from build123d import *

# Parameters (mm, degrees)
F0_W     = 150
F0_H     = 150
F1_DEPTH = 2


with BuildPart() as f1:
    # F0 (on Front) → F1 (new body)
    with BuildSketch(Plane.XZ):
        Rectangle(F0_W, F0_H)
        with BuildLine():
            ThreePointArc((-46.568542, -56.568542), (-65.807338, -60.395377), (-49.497475, -49.497475))
            ThreePointArc((-49.497475, -49.497475), (-47.329747, -52.741708), (-46.568542, -56.568542))
        make_face(mode=Mode.SUBTRACT)
        with BuildLine():
            ThreePointArc((66.568542, -56.568542), (52.741708, -65.807338), (49.497475, -49.497475))
            ThreePointArc((49.497475, -49.497475), (60.395377, -47.329747), (66.568542, -56.568542))
        make_face(mode=Mode.SUBTRACT)
        with BuildLine():
            ThreePointArc((-46.568542, 56.568542), (-47.329747, 52.741708), (-49.497475, 49.497475))
            ThreePointArc((-49.497475, 49.497475), (-65.807338, 60.395377), (-46.568542, 56.568542))
        make_face(mode=Mode.SUBTRACT)
        with BuildLine():
            ThreePointArc((-28.284271, 28.284271), (0, 40), (28.284271, 28.284271))
            ThreePointArc((28.284271, 28.284271), (36.955181, 15.307337), (40, 0))
            ThreePointArc((40, 0), (36.955181, -15.307337), (28.284271, -28.284271))
            ThreePointArc((28.284271, -28.284271), (0, -40), (-28.284271, -28.284271))
            ThreePointArc((-28.284271, -28.284271), (-40, 0), (-28.284271, 28.284271))
        make_face(mode=Mode.SUBTRACT)
        with BuildLine():
            ThreePointArc((66.568542, 56.568542), (60.395377, 47.329747), (49.497475, 49.497475))
            ThreePointArc((49.497475, 49.497475), (52.741708, 65.807338), (66.568542, 56.568542))
        make_face(mode=Mode.SUBTRACT)
    extrude(amount=F1_DEPTH)


solid = f1.part
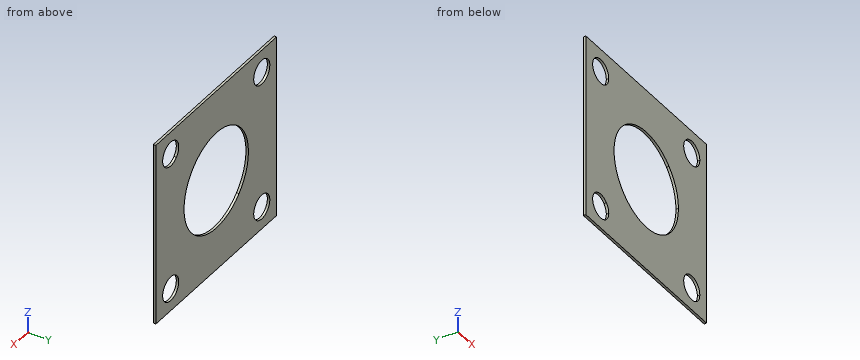
Could you check a few things on this model? Use its own coordinates, in mm. Give positions to 0.01 mm unless a question says otherwise; leave off trailing zeros. Order: outer loops, then holes, each group sorted by start corner. A loop starts at its lowest first (then second) coordinate and runs counter-clockwise, first axis right, second up. Notation, with made-up numbers: (16.5, 59.5) -> (47.5, 59.5) arc R22 cw to (47.5, 88.5) -> close; hole circle Ø3 at (32, 29.5). An arc over 180 degrees is marked (long way). Answer in a Markdown table with one row per item. Add a question column.
Item 1: Imagine slicing it at D-D (x = -60.5). List the corners of the cut face in (y, z) for me, and give its area (3 significant figures).
Item 2: Imagine slicing it at A-A (y = -0.55). List the corners of the cut face in (x, z) for me.
Item 3: Please list where these lines run through material, in increasing order: probe 1 along Z at (x, y) = (58, -1); probe 2 along X at (y, z) = (-1.3, -47.5); probe 3 along X at (y, z) = (-1.2, 63).
Item 4: I'm going to push a flat-ended pin straight in: P1, Ø18, axis at x = 56.57, z = 56.57, coming from the +Y side. Where does the tip first touch, or does it pass through?
Item 5: Imagine slicing it at B-B (x = 37.5). List the corners of the cut face in (y, z) for me, and give its area (3 significant figures).
Item 6: Imagine slicing it at C-C (z = 37.5). List the corners of the cut face in (x, y) for me.
Result:
| question | item | result |
|---|---|---|
| 1 | outline | (-2, -75) -> (0, -75) -> (0, -65.76) -> (-2, -65.76) -> close; (-2, -47.37) -> (0, -47.37) -> (0, 47.37) -> (-2, 47.37) -> close; (-2, 65.76) -> (0, 65.76) -> (0, 75) -> (-2, 75) -> close |
| 1 | area | 226 mm2 |
| 2 | outline | (-75, -75) -> (75, -75) -> (75, 75) -> (-75, 75) -> close; hole (-49.5, -49.5) arc R10 ccw (long way) to (-46.57, -56.57) arc R10 ccw to start; hole (-49.5, 49.5) arc R10 ccw to (-46.57, 56.57) arc R10 ccw (long way) to start; hole (-28.28, -28.28) arc R40 ccw to (28.28, -28.28) arc R40 ccw to (40, 0) arc R40 ccw to (28.28, 28.28) arc R40 ccw to (-28.28, 28.28) arc R40 ccw to start; hole (49.5, -49.5) arc R10 ccw (long way) to (66.57, -56.57) arc R10 ccw to start; hole (49.5, 49.5) arc R10 ccw to (66.57, 56.57) arc R10 ccw (long way) to start |
| 3 | probe 1 | -75 to -66.47, -46.67 to 46.67, 66.47 to 75 |
| 3 | probe 2 | -75 to -60.78, -52.35 to 52.35, 60.78 to 75 |
| 3 | probe 3 | -75 to -64.23, -48.91 to 48.91, 64.23 to 75 |
| 4 | P1 | through |
| 5 | outline | (-2, -75) -> (0, -75) -> (0, -13.92) -> (-2, -13.92) -> close; (-2, 13.92) -> (0, 13.92) -> (0, 75) -> (-2, 75) -> close |
| 5 | area | 244 mm2 |
| 6 | outline | (-75, -2) -> (-13.92, -2) -> (-13.92, 0) -> (-75, 0) -> close; (13.92, -2) -> (75, -2) -> (75, 0) -> (13.92, 0) -> close |
